For this review, take the finished solid that the model builds, in its own axes (mm). Face numbers are marked on the shaded views. A direction names the side the tool comes from. Give positions to 0.01 mm unless a question says otherwise; leave off trailing zeros. Loops run counter-clockwise (first coordinate to the right, second up) from the corner with the lowest first, then second, coordinate; pieces in that order, holes last. Notation, with made-up numbers: (-20.75, -29.75) -> (6.25, -29.75) arc R32 cw to (6.25, 9.25) -> close; hole circle Ø11 at (1, 16.25). An arc over 180 degrees is marked (long way). Write each question's results on one line, items separated by ' | '. Start each with the question number.
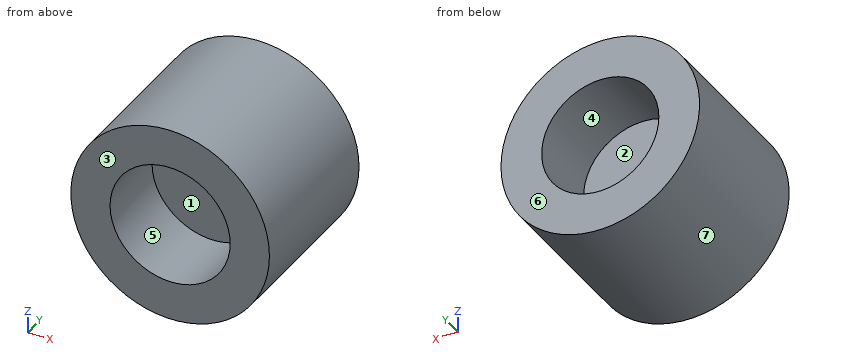
```python
from build123d import *

# Parameters (mm, degrees)
F0_R     = 127
F1_DEPTH = 203.2
F2_R     = 76.870137
F3_DEPTH = 95.25
F4_R     = 74.972923
F5_DEPTH = 95.25


with BuildPart() as f1:
    # F0 (on Front) → F1 (new body)
    with BuildSketch(Plane.XZ):
        Circle(F0_R)
    extrude(amount=-F1_DEPTH)

    # F2 (on face) → F3 (cut)
    with BuildSketch(Plane.XZ):
        Circle(F2_R)
    extrude(amount=-F3_DEPTH, mode=Mode.SUBTRACT)

    # F4 (on face) → F5 (cut)
    with BuildSketch(Plane(origin=(0, 203.2, 0), x_dir=(-1, 0, 0), z_dir=(0, 1, 0))):
        Circle(F4_R)
    extrude(amount=-F5_DEPTH, mode=Mode.SUBTRACT)


solid = f1.part
```
1. We need section A-A (z = 0). Write out the cut boundary in (x, y), plus the area to 3 significant figures.
2. Machinability: for the marked faces 1, 2 and 3, which of the approach directions +Z, -Z, +X, -X, +Y, -Y give a long, thin tool a straight path to every point of the face, cutting with its end or side? Answer none if there is none.
3. Wall thickness on L1, parallel to Z at x = 0, y = 24.5; L2, parallel to Z at x = 0, y = 177; L3, parallel to Y at x = -45, z = 1.5: over which ranges is each line inside the solid? List them lowest first.
4. For pin 1 Ø1 at (x, y) = (-12.5, 135) entering from -Z; pin 2 Ø5 at (x, y) = (-92.5, 128.5) entering from -Z; pin 3 Ø6 at (y, z) = (166, -6) entering from -X; pin 4 Ø10 at (x, z) = (-90.5, 28.5) entering from -Y, all flat-tipped, find the tip position at first contact; note any pin that passes through.
5. We need section D-D (y = 103). Write out the cut boundary in (x, z), plus the area to 3 significant figures.
6. We need section C-C (y = 175). Write out the cut boundary in (x, z).
7. We need section B-B (x = 0). Write out the cut boundary in (y, z), plus the area to 3 significant figures.
8. Draft analysis for pull direction X (two halves, no side actions). For the marked faces 4, 5, 6 and 7, state which applies: released by +X, released by -X, zero draft, split by the parting line, or undercut.
Response:
1) outline: (-127, 0) -> (-76.87, 0) -> (-76.87, 95.25) -> (76.87, 95.25) -> (76.87, 0) -> (127, 0) -> (127, 203.2) -> (74.97, 203.2) -> (74.97, 107.95) -> (-74.97, 107.95) -> (-74.97, 203.2) -> (-127, 203.2) -> close | area: 22,700 mm2
2) face 1: -Y | face 2: +Y | face 3: +Z, -Z, +X, -X, -Y
3) L1: z = -127 to -76.87, 76.87 to 127 | L2: z = -127 to -74.97, 74.97 to 127 | L3: y = 95.25 to 107.95
4) pin 1: stops at z = -126.43 | pin 2: stops at z = -89.6 | pin 3: stops at x = -126.96 | pin 4: stops at y = 0
5) outline: circle Ø254 at (0, 0) | area: 50,700 mm2
6) outline: circle Ø254 at (0, 0); hole circle Ø149.95 at (0, 0)
7) outline: (0, -127) -> (203.2, -127) -> (203.2, -74.97) -> (107.95, -74.97) -> (107.95, 74.97) -> (203.2, 74.97) -> (203.2, 127) -> (0, 127) -> (0, 76.87) -> (95.25, 76.87) -> (95.25, -76.87) -> (0, -76.87) -> close | area: 22,700 mm2
8) face 4: undercut | face 5: undercut | face 6: zero draft | face 7: split by the parting line
